Check sheet for the drawn part. Datum: minimum x, y, z corner. Units: mm. Give positions to 0.01 mm unless a question says otherwise; leave off trailing zeros. Write each loop counter-clockwise with the first axis right and the second up, starting at its lowest first coordinate (ties: lowest second). Pieces come first, ordered by that corner, then holes. Notation, with made-up numbers: M 62,-27.75 L 107,-27.75 A21 ccw 107,-19.75 Z; hole C -23.5,47 d3. An arc over 180 degrees is marked long. Write item = value, one per line. Start each with the question number.
1) Sectioned sample at A-A, the plane y = 20.25. Record the cut outline in (x, z).
2) Sectioned sample at B-B, the plane z = 6.5. Record the cut outline in (x, y).
3) Sectioned sample at C-C, the plane x = 104.5. Record the cut outline in (y, z), then the cut area to 3 significant figures.
4) Gauge pin test, flat ends, axial feed: pin 1 (2 mm diameter, centred on x = 115.5, y = 10, fed in from +Z); pin 2 (5 mm diameter, centred on y = 11, z = 49, fed in from +X). Record the tip position at first contact, or that the pin passes through.
5) Scan lines: L1, parallel to X at y = 23, z = 65; L2, parallel to X at y = 12.25, z = 73; L3, parallel to Z at x = 113.5, y = 7.75. Record each from-to range of solid material in increasing order.
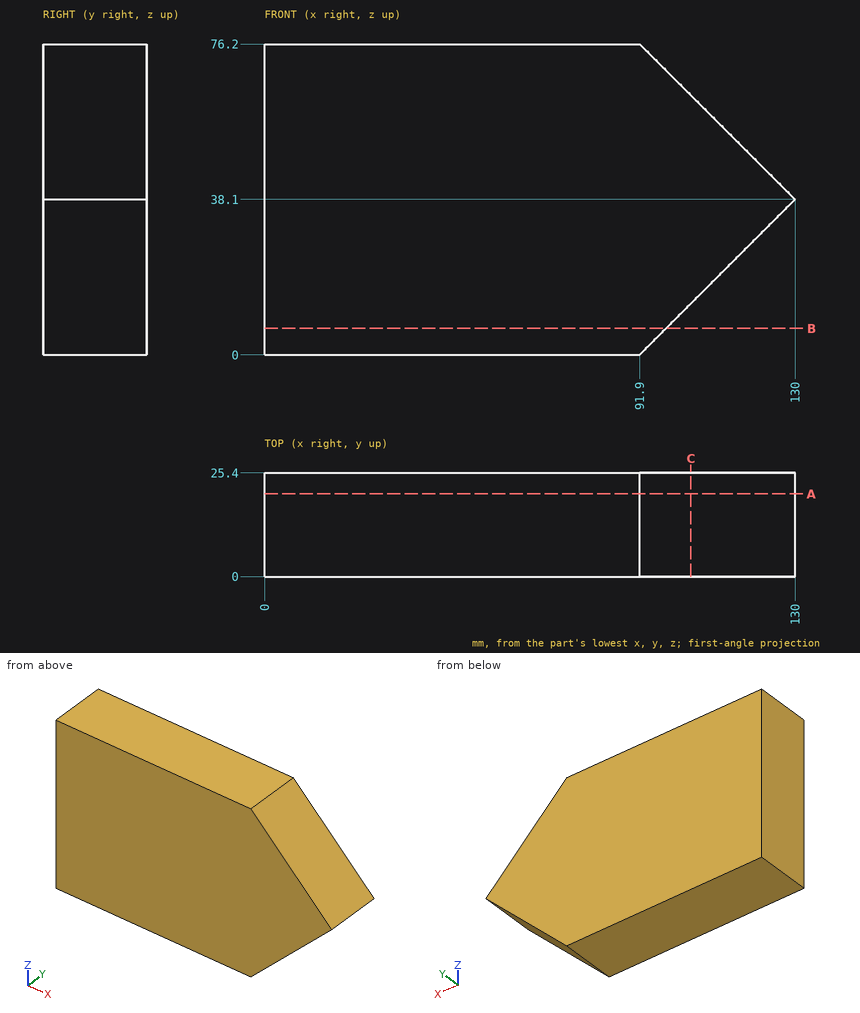
Data:
q1.outline = M 0,0 L 91.9,0 L 130,38.1 L 91.9,76.2 L 0,76.2 Z
q2.outline = M 0,0 L 98.4,0 L 98.4,25.4 L 0,25.4 Z
q3.outline = M 0,12.6 L 25.4,12.6 L 25.4,63.6 L 0,63.6 Z
q3.area = 1,300 mm2
q4.pin_1 = 53.6
q4.pin_2 = 121.6
q5.L1 = 0 to 103.1
q5.L2 = 0 to 95.1
q5.L3 = 21.6 to 54.6
